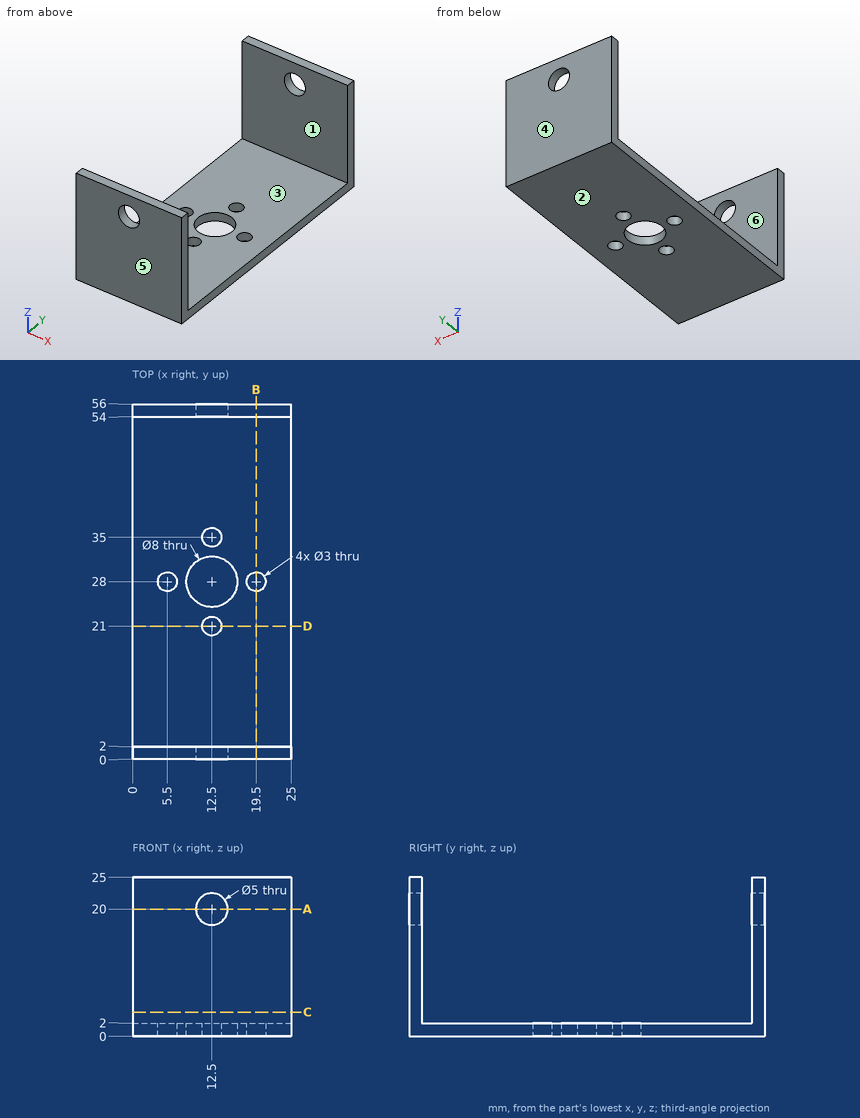
Answer from the drawing. Dimensions are ordinates in mm from the lowest x, y and z of the part. A direction names the side the tool comes from. Give positions to 0.01 mm unless a question says otherwise; leave off trailing zeros. Write each loop counter-clockwise with the first axis right and the second up, starting at its lowest first coordinate (ties: lowest second). Pieces come first, ordered by that corner, then holes. Notation, with made-up numbers: (11, -15) -> (17, -15) arc R25 cw to (17, -3) -> close; hole circle Ø10 at (41, 61). An arc over 180 degrees is marked (long way). One line per question, with ' | ' between items. Start each with the question number.
1. Section D-D (y = 21) is taken. Determine the outline of the cut face in (x, z).
2. For a pull along Y with two mould halves and no side action, classify the marked faces 3, 4, 5 and 6 as pulls with the +Y half, pulls with the -Y half, needs draft (parallel to the pull), parting line crosses it, or undercut.
3. Section B-B (x = 19.5) is taken. Determine the outline of the cut face in (y, z).
4. For the marked faces 1 and 2, determine the directions among +Z, -Z, +X, -X, +Y, -Y from which every point of the face is accessible in a straight line to the end or side of a thin tool.
5. Find the intervals of material crossed by probe 1 along Y at (x, z) = (12.5, 1.35); probe 2 along Y at (x, z) = (17, 4); probe 3 along Y at (x, z) = (5.5, 1), in increasing order.
6. Given pin 1 Ø8 at (x, y) = (5.5, 9) entering from +Z, flat-ended and moving along its own axis, determine where the tip first touches the part or whether it passes through.
7. Section A-A (z = 20) is taken. Determine the outline of the cut face in (x, y).
8. Section C-C (z = 3.75) is taken. Determine the outline of the cut face in (x, y).
Response values:
1) outline: (0, 0) -> (11, 0) -> (11, 2) -> (0, 2) -> close; (14, 0) -> (25, 0) -> (25, 2) -> (14, 2) -> close
2) face 3: undercut | face 4: pulls with the +Y half | face 5: pulls with the -Y half | face 6: undercut
3) outline: (0, 0) -> (26.5, 0) -> (26.5, 2) -> (2, 2) -> (2, 25) -> (0, 25) -> close; (29.5, 0) -> (56, 0) -> (56, 25) -> (54, 25) -> (54, 2) -> (29.5, 2) -> close
4) face 1: +Z, +X, -X | face 2: -Z, +X, -X, +Y, -Y
5) probe 1: 0 to 19.5, 22.5 to 24, 32 to 33.5, 36.5 to 56 | probe 2: 0 to 2, 54 to 56 | probe 3: 0 to 26.5, 29.5 to 56
6) pin 1: z = 2
7) outline: (0, 0) -> (10, 0) -> (10, 2) -> (0, 2) -> close; (0, 54) -> (10, 54) -> (10, 56) -> (0, 56) -> close; (15, 0) -> (25, 0) -> (25, 2) -> (15, 2) -> close; (15, 54) -> (25, 54) -> (25, 56) -> (15, 56) -> close
8) outline: (0, 0) -> (25, 0) -> (25, 2) -> (0, 2) -> close; (0, 54) -> (25, 54) -> (25, 56) -> (0, 56) -> close
